Design review of the part built by this model. Coordinates are the model's own, in mm. A direction names the side the tool comes from. Coordinates: 2 decimals unless noted, no trailing zeros. Loops run counter-clockwise (first coordinate to the right, second up) from the corner with the lowest first, then second, coordinate; pieces in that order, holes last. Notation, with made-up numbers: (14.25, 50) -> (52.25, 50) arc R25 cw to (52.25, 85) -> close; hole circle Ø1 at (55.25, -1.5). An arc over 180 degrees is marked (long way). Answer as a JSON object with one key per item and string values.
```python
from build123d import *

# Parameters (mm, degrees)
F1_DEPTH = 63.5
F2_DEPTH = 7.9375
F4_R     = 7.62


with BuildPart() as f1:
    # F0 (on Front) → F1 (new body, symmetric)
    with BuildSketch(Plane.XZ):
        Polygon((-41.275, -9.525), (41.275, -9.525), (41.275, 9.525), (25.4, 9.525), (-41.275, 9.525), align=None)
    extrude(amount=F1_DEPTH, both=True)

    # F0 (on Front) → F2 (join, symmetric)
    with BuildSketch(Plane.XZ):
        with BuildLine():
            add(Edge.make_bspline(
                [(-41.275, 9.525), (-27.703339234, 32.6747409999), (3.8328881679, 53.8919653869), (49.2122638223, 57.7419443287)],
                knots=[0, 0, 0, 0, 102.5320371125, 102.5320371125, 102.5320371125, 102.5320371125], degree=3))
            Line((-41.275, 9.525), (25.4, 9.525))
            Line((25.4, 9.525), (25.4, 27.0002))
            ThreePointArc((25.4, 27.0002), (32.0493463866, 46.4429284139), (49.2122638223, 57.7419443287))
        make_face()
        with BuildLine():
            Line((25.4, 9.525), (41.275, 9.525))
            Line((41.275, 9.525), (41.275, 27.0002))
            ThreePointArc((41.275, 27.0002), (43.4017785364, 34.9375819102), (49.2122638223, 40.7482169251))
            Line((49.2122638223, 40.7482169251), (49.2122638223, 57.7419443287))
            ThreePointArc((49.2122638223, 57.7419443287), (32.0493463866, 46.4429284139), (25.4, 27.0002))
            Line((25.4, 27.0002), (25.4, 9.525))
        make_face()
        with BuildLine():
            ThreePointArc((57.15, 58.7502), (53.149242724, 58.4971274885), (49.2122638223, 57.7419443287))
            Line((49.2122638223, 57.7419443287), (49.2122638223, 40.7482169251))
            ThreePointArc((49.2122638223, 40.7482169251), (53.0411159475, 42.3342371997), (57.15, 42.8752))
            Line((57.15, 42.8752), (74.6156958322, 42.8752))
            Line((74.6156958322, 42.8752), (74.6271054395, 58.7502))
            Line((74.6271054395, 58.7502), (57.15, 58.7502))
        make_face()
    extrude(amount=F2_DEPTH, both=True)

    # F0 (on Front) → F3 (revolve)
    with BuildSketch(Plane.XZ):
        Polygon((100.0122638223, 66.675), (74.6328011155, 66.675), (74.6271054395, 58.7502), (74.6156958322, 42.8752), (74.6122638223, 38.1), (100.0122638223, 38.1), align=None)
    revolve(axis=Axis((74.6225324689, 0, 52.3875), (0.0007187152, 0, 0.9999997417)))

    # F4
    f4_edges = [f1.edges().sort_by_distance(p)[0] for p in [
        (41.275, -63.5, 0),
        (-41.275, -63.5, 0),
        (41.275, 63.5, 0),
        (-41.275, 63.5, 0),
    ]]
    fillet(f4_edges, radius=F4_R)


solid = f1.part
```
1) For faces 4 (the flat face through (15, 7.938, 29)), 5 (the flat face through (41.275, -1, 0)), 6 (the flat face through (1, -36, 9.525)), list the 3-axis set-ups (+Z, -Z, +X, -X, +Y, -Y) from which the entire face can be reached by the end or side of a thin tool; tool diameter is ignored.
Completed:
{"face 4": "+Z, -X, +Y", "face 5": "-Z, +X, +Y, -Y", "face 6": "+Z, +X, -X, -Y"}
2) The part is to be moulded in two halves that separate along X. For faces 1 (the cylindrical face through (-38.98, 61.33, -0.13)), 2 (the cylindrical face through (43.71, -0.11, 35.45)), 3 (the flat face through (15, -7.938, 29)), say which applies: pulls with the +X half, pulls with the -X half, needs draft (parallel to the pull), parting line crosses it, or undercut.
Completed:
{"face 1": "pulls with the -X half", "face 2": "undercut", "face 3": "needs draft"}
3) Add section A-A, the plane z = 3. Give the boundary of the cut face in (x, y) (3 decimals), and give its area (3 significant figures).
Completed:
{"outline": "(-41.275, -55.88) arc R7.62 ccw to (-33.655, -63.5) -> (33.655, -63.5) arc R7.62 ccw to (41.275, -55.88) -> (41.275, 55.88) arc R7.62 ccw to (33.655, 63.5) -> (-33.655, 63.5) arc R7.62 ccw to (-41.275, 55.88) -> close", "area": "10,400 mm²"}
4) Clearance check with flat-ended pins moving along their axes: pin 1 Ø24.5 at (x, z) = (10.5, 43) entering from +Y; pin 2 Ø10 at (y, z) = (-20.5, 39) entering from +X; pin 3 Ø6 at (y, z) = (-10.5, 23.5) entering from -X. State where each tip first meets the part, or that it passes through.
Completed:
{"pin 1": "y = 7.94", "pin 2": "x = 94.73", "pin 3": "x = -32.05"}
5) Add section B-B, the plane y = -51. Give the boundary of the cut face in (x, z) (3 decimals), and give its area (3 significant figures).
Completed:
{"outline": "(-41.275, -9.525) -> (41.275, -9.525) -> (41.275, 9.525) -> (-41.275, 9.525) -> close", "area": "1,570 mm²"}
6) Wall thickness on probe 1 along Y at (x, z) = (30, 51); probe 2 along Z at (x, y) = (-3.5, -31) (3 decimals); probe 3 along X at (y, z) = (-39.5, -5.5) (3 decimals): over which ranges is each line inside the solid? List them lowest first.
Completed:
{"probe 1": "-7.94 to 7.94", "probe 2": "-9.525 to 9.525", "probe 3": "-41.275 to 41.275"}
